```python
from build123d import *

# Parameters (mm, degrees)
SKETCH005_R      = 7
EXTRUDE005_DEPTH = 10
EXTRUDE004_DEPTH = 800


with BuildPart() as extrude001:
    # Sketch005 (on Face1 of Extrude004) → Extrude005 (new body)
    with BuildSketch(Plane.XZ):
        with Locations((-700, -40.447773)):
            Circle(SKETCH005_R)
        with Locations((700, -39.622757)):
            Circle(SKETCH005_R)
        with Locations((-500, -40.447773)):
            Circle(SKETCH005_R)
        with Locations((-299.49234, -40.447773)):
            Circle(SKETCH005_R)
        with Locations((-99.23851, -40.447773)):
            Circle(SKETCH005_R)
        with Locations((101.01532, -40.447773)):
            Circle(SKETCH005_R)
        with Locations((301.26915, -40.447773)):
            Circle(SKETCH005_R)
        with Locations((501.52298, -40.447773)):
            Circle(SKETCH005_R)
    extrude(amount=-EXTRUDE005_DEPTH)


with BuildPart() as angle:
    # AngleSteel006 → Extrude004 (new body, symmetric)
    with BuildSketch(Plane(origin=(0, 20.5898499587, -20.5898499587), x_dir=(0, -1, 0), z_dir=(1, 0, 0))):
        with BuildLine():
            Line((20.5898499587, -20.5898499587), (20.5898499587, 54.4101500413))
            Line((20.5898499587, 54.4101500413), (18.5898499587, 54.4101500413))
            ThreePointArc((18.5898499587, 54.4101500413), (15.761422834, 53.238577166), (14.5898499587, 50.4101500413))
            Line((14.5898499587, 50.4101500413), (14.5898499587, -6.0898499587))
            ThreePointArc((14.5898499587, -6.0898499587), (12.1002575988, -12.1002575988), (6.0898499587, -14.5898499587))
            Line((6.0898499587, -14.5898499587), (-50.4101500413, -14.5898499587))
            ThreePointArc((-50.4101500413, -14.5898499587), (-53.238577166, -15.761422834), (-54.4101500413, -18.5898499587))
            Line((-54.4101500413, -18.5898499587), (-54.4101500413, -20.5898499587))
            Line((-54.4101500413, -20.5898499587), (20.5898499587, -20.5898499587))
        make_face()
    extrude(amount=EXTRUDE004_DEPTH, both=True)

    # Cut002: cut Extrude001
    add(extrude001.part, mode=Mode.SUBTRACT)


solid = angle.part
```
Verification items for the finished model (mm, model axes). A direction names the side the tool comes from. Coordinates: 2 decimals unless noted, no trailing zeros. Loops run counter-clockwise (first coordinate to the right, second up) from the corner with the lowest first, then second, coordinate; pieces in that order, holes last. Notation, with made-up numbers: (6, 39.5) - (27, 39.5) arc R32 cw to (27, 65.5) - close; hole circle Ø11 at (-1, 63.25). An arc over 180 degrees is marked (long way). Return JSON: item names as keys, results as strings.
1. Go/stop test with flat-tipped pins: pin 1 (1.5 mm diameter, centred on x = -25.5, z = -47.5, fed in from +Y); pin 2 (12.5 mm diameter, centred on x = 101.02, z = -40.45, fed in from +Y); pin 3 (1 mm diameter, centred on x = 266.5, y = 66, fed in from -Z). Record where each tip stops, or that it passes through.
Established:
{"pin 1": "stops at y = 6", "pin 2": "passes through", "pin 3": "stops at z = -6"}
2. Section check A-A, the plane x = -131.5. Record the boundary of the cut face in (y, z).
Established:
{"outline": "(0, -75) - (2, -75) arc R4 ccw to (6, -71) - (6, -14.5) arc R8.5 cw to (14.5, -6) - (71, -6) arc R4 ccw to (75, -2) - (75, 0) - (0, 0) - close"}
3. Section check B-B, the plane y = 57. Record the boundary of the cut face in (x, z), then the cut area to 3 significant figures.
Established:
{"outline": "(-800, -6) - (800, -6) - (800, 0) - (-800, 0) - close", "area": "9,600 mm2"}
4. Tool access check on faces 1 (the flat face through (11, 38, 0)), 2 (the flat face through (11, 6, -43)). Record the directions out of +Z, -Z, +X, -X, +Y, -Y that give a thin tool (end or side, any length) a straight path to the whole face; none if there is none.
Established:
{"face 1": "+Z, +X, -X, +Y, -Y", "face 2": "-Z, +X, -X, +Y"}
5. Thickness scan on L1, parallel to Z at x = -500, y = 3; L2, parallel to Z at x = 679.5, y = 23; L3, parallel to Y at x = 408, z = -17. Record the ranges inside material, lowest first.
Established:
{"L1": "z = -74.87 to -47.45, -33.45 to 0", "L2": "z = -6 to 0", "L3": "y = 0 to 6"}
